from build123d import *

# Parameters (mm, degrees)
F1_DEPTH = 18.288
F2_T     = -177.8
F3_T     = -2.54


with BuildPart() as f1:
    # F0 (on Top) → F1 (new body)
    with BuildSketch(Plane.XY):
        Polygon((5.212843, 44.114474), (-14.399178, 41.653003), (-30.152951, 29.715296), (-37.827265, 11.500053), (-35.365794, -8.111968), (-23.428087, -23.865741), (-5.212843, -31.540055), (14.399178, -29.078584), (30.152951, -17.140877), (37.827265, 1.074367), (35.365794, 20.686388), (23.428087, 36.44016), align=None)
    extrude(amount=F1_DEPTH)

    # F2
    f2_openings = [f1.faces().sort_by_distance(p)[0] for p in [
        (0, 6.28721, 18.288),
    ]]
    offset(amount=F2_T, openings=f2_openings)

    # F3
    f3_openings = [f1.faces().sort_by_distance(p)[0] for p in [
        (0, 6.28721, 18.288),
    ]]
    offset(amount=F3_T, openings=f3_openings)


solid = f1.part
Build history of the part. All positions in model axes, mm. A direction names the side the tool comes from. Round coordinates to 2 decimals unless told otherwise and drop trailing zeros. Loops run counter-clockwise (first coordinate to the right, second up) from the corner with the lowest first, then second, coordinate; pieces in that order, holes last. Notation, with made-up numbers: (31.25, -27.75) -> (59.25, -27.75) arc R19 cw to (59.25, -15.75) -> close; hole circle Ø2 at (67.25, -39.75). An arc over 180 degrees is marked (long way). One line per item, written item: value. Start each with the question number.
Q1. Cut at A-A on z = 10.5. List the corners of the cut face in (x, y), plus the area to 3 significant figures.
Q2. Two-plate mould, pull along X, no slides. Class faces 1 (the face through (4.456, -30.327, 9.016)), 2 (the face through (31, -10, 18.288)), 3 (the face through (-20.639, 33.738, 10.304)): released by +X, released by -X, zero draft, split by the parting line, or undercut.
Q3. Cut at B-B on y = 14.5. List the corners of the cut face in (x, z).
Q4. Drop flat-ended pins along their axis: pin 1 Ø5 at (x, z) = (-1.5, 10) entering from -Y; pin 2 Ø1 at (x, z) = (24, 9) entering from -Y; pin 3 Ø2 at (y, z) = (33, 2) entering from +X. Give the stop position or say it passes through.
Q5. 3-axis set-ups, long thin cutter, end or side, ignore diameter. For faces 4 (the face through (-34.092, 2.138, 10.304)), 5 (the face through (-22.166, 35.768, 9.016)): which of +Z, -Z, +X, -X, +Y, -Y reach the whole face in a straight line?
Q6. Cut at C-C on x = -15.5. List the corners of the cut face in (y, z).
Q7. Probe line 1 along Z through (x, y) = (2.5, 29); line 2 along Y through (x, z) = (20.5, 5); line 3 along X through (y, z) = (-26, 4.25). List the from-to ranges inside material, lowest first.
Computed:
1. outline: (-37.83, 11.5) -> (-35.37, -8.11) -> (-23.43, -23.87) -> (-5.21, -31.54) -> (14.4, -29.08) -> (30.15, -17.14) -> (37.83, 1.07) -> (35.37, 20.69) -> (23.43, 36.44) -> (5.21, 44.11) -> (-14.4, 41.65) -> (-30.15, 29.72) -> close; hole (-35.22, 11.14) -> (-32.93, -7.12) -> (-21.81, -21.79) -> (-4.85, -28.94) -> (13.41, -26.64) -> (28.08, -15.53) -> (35.22, 1.43) -> (32.93, 19.69) -> (21.81, 34.36) -> (4.85, 41.51) -> (-13.41, 39.22) -> (-28.08, 28.1) -> close
1. area: 582 mm²
2. face 1: released by +X
2. face 2: zero draft
2. face 3: undercut
3. outline: (-36.56, 0) -> (36.14, 0) -> (36.14, 18.29) -> (33.58, 18.29) -> (33.58, 2.54) -> (-33.81, 2.54) -> (-33.81, 18.29) -> (-36.56, 18.29) -> close
4. pin 1: y = -31.39
4. pin 2: y = -22.18
4. pin 3: x = 26.79
5. face 4: +Z
5. face 5: +Z, -Z, -X, +Y
6. outline: (-27.21, 0) -> (40.82, 0) -> (40.82, 18.29) -> (37.63, 18.29) -> (37.63, 2.54) -> (-24.45, 2.54) -> (-24.45, 18.29) -> (-27.21, 18.29) -> close
7. line 1: 0 to 2.54
7. line 2: -24.46 to -21.27, 34.92 to 37.67
7. line 3: -18.36 to -11.82, 14.26 to 18.46
